from build123d import *

# Parameters (mm, degrees)
ESQUISSE2_R             = 3
ESQUISSE2_R_2           = 1.825
BOSS_EXTRU_1_DEPTH      = 11.5
ESQUISSE3_R             = 10
ENL_V_MAT_EXTRU_1_DEPTH = 4
CONG_1_R                = 5
FILLET1_R               = 5


with BuildPart() as part:
    # Esquisse2 → Boss.-Extru.1 (new body)
    # profile 1 of 4: a face of its own
    with BuildSketch(Plane.XY):
        with Locations((-10, 5)):
            Circle(ESQUISSE2_R)
        with Locations((-10, 5)):
            Circle(ESQUISSE2_R_2, mode=Mode.SUBTRACT)
    # profile 2 of 4: a face of its own
    with BuildSketch(Plane.XY):
        with Locations((10, 5)):
            Circle(ESQUISSE2_R)
        with Locations((10, 5)):
            Circle(ESQUISSE2_R_2, mode=Mode.SUBTRACT)
    # profile 3 of 4: a face of its own
    with BuildSketch(Plane.XY):
        with Locations((0, -6.825)):
            Circle(ESQUISSE2_R)
        with Locations((0, -6.825)):
            Circle(ESQUISSE2_R_2, mode=Mode.SUBTRACT)
    # profile 4 of 4: a face of its own
    with BuildSketch(Plane.XY):
        Polygon((-8.175, 5), (8.175, 5), (0, -5), align=None)
    extrude(amount=BOSS_EXTRU_1_DEPTH)

    # Esquisse3 → Enlèv. mat.-Extru.1 (cut)
    with BuildSketch(Plane.XY.offset(3.75)):
        with Locations((10, 5)):
            Circle(ESQUISSE3_R)
    extrude(amount=ENL_V_MAT_EXTRU_1_DEPTH, mode=Mode.SUBTRACT)

    # Congé1
    # the kernel refuses this fillet: 5 mm, written as the material it adds along each edge
    with BuildSketch(Plane(origin=(-7, 5, 0), x_dir=(-0.3311912213512006, 0.9435636570469954, 0), z_dir=(0, 0, 1))) as cong_1_piece_1:
        with BuildLine():
            CenterArc((3.643103435, -4.717818285), CONG_1_R, 109.341093727, 51.317812547)
            Line((-1.07471485, -3.061862178), (0, 0))
            ThreePointArc((0, 0), (0.993573664, -0.169309029), (1.987147328, 0))
        make_face()
    extrude(amount=11.5)
    with BuildSketch(Plane(origin=(-7.231093941, 3.845374851, 11.5), x_dir=(-0.7661000074497634, -0.6427213848826507, 0), z_dir=(0, 0, -1))) as cong_1_piece_2:
        with BuildLine():
            CenterArc((5.056907819, -4.440322454), CONG_1_R, 117.368969646, 63.360078756)
            Line((0.057312583, -4.503942212), (0, 0))
            ThreePointArc((0, 0), (1.379156678, -0.335806528), (2.758313356, 0))
        make_face()
    extrude(amount=11.5)
    with BuildSketch(Plane(origin=(-0.858096974, -3.950340093, 11.5), x_dir=(-0.6329215353519139, 0.7742159453846039, 0), z_dir=(0, 0, -1))) as cong_1_piece_3:
        with BuildLine():
            CenterArc((4.246739065, -5), CONG_1_R, 90, 61.27443838)
            ThreePointArc((-0.137920096, -2.596926126), (0.227062491, -1.314184518), (0, 0))
            Line((0, 0), (4.246739065, 0))
        make_face()
    extrude(amount=11.5)
    with BuildSketch(Plane(origin=(7.231093941, 3.845374851, 11.5), x_dir=(-0.6329215353519138, -0.774215945384604, 0), z_dir=(0, 0, -1))) as cong_1_piece_4:
        with BuildLine():
            CenterArc((4.504306848, -5), CONG_1_R, 90, 63.360078756)
            ThreePointArc((0.035096646, -2.758090063), (0.353327666, -1.374772245), (0, 0))
            Line((0, 0), (4.504306848, 0))
        make_face()
    extrude(amount=3.75)
    with BuildSketch(Plane(origin=(7, 5, 11.5), x_dir=(-1, 0, 0), z_dir=(0, 0, -1))) as cong_1_piece_5:
        with BuildLine():
            CenterArc((3.244997998, 5), CONG_1_R, 218.682187453, 51.317812547)
            ThreePointArc((-0.658125751, 1.875), (-0.169309029, 0.993573664), (0, 0))
            Line((0, 0), (3.244997998, 0))
        make_face()
    extrude(amount=3.75)
    with BuildSketch(Plane(origin=(0.858096974, -3.950340093, 11.5), x_dir=(0.7395598752725667, -0.6730907746261462, 0), z_dir=(0, 0, -1))) as cong_1_piece_6_section:
        with BuildLine():
            CenterArc((4.767740899, -4.505933799), CONG_1_R, 115.685497342, 61.27443838)
            Line((-0.225222573, -4.240762606), (0, 0))
            ThreePointArc((0, 0), (1.300292973, -0.29643972), (2.600585945, 0))
        make_face()
    cong_1_piece_6 = extrude(amount=11.5, mode=Mode.PRIVATE)
    cong_1_piece_6 = cong_1_piece_6 - Plane(origin=(10, 5, 9.625), x_dir=(1, 0, 0), z_dir=(0, 0, -1)) * Cylinder(10, 40, mode=Mode.PRIVATE)
    add(cong_1_piece_6)
    with BuildSketch(Plane(origin=(0.858096974, -3.950340093, 11.5), x_dir=(0.7395598752725667, -0.6730907746261462, 0), z_dir=(0, 0, -1))) as cong_1_piece_7_section:
        with BuildLine():
            CenterArc((4.767740899, -4.505933799), CONG_1_R, 115.685497342, 61.27443838)
            Line((-0.225222573, -4.240762606), (0, 0))
            ThreePointArc((0, 0), (1.300292973, -0.29643972), (2.600585945, 0))
        make_face()
    cong_1_piece_7 = extrude(amount=22.116847663, mode=Mode.PRIVATE)
    cong_1_piece_7 = split(cong_1_piece_7, bisect_by=Plane(origin=(2.909028405, -1.544063306, 7.75), z_dir=(0, 0, 1)), keep=Keep.TOP, mode=Mode.PRIVATE)
    add(cong_1_piece_7)
    with BuildSketch(Plane(origin=(0.858096974, -3.950340093, 22.116847663), x_dir=(0.7395598752725666, -0.6730907746261463, 0), z_dir=(0, 0, -1))) as cong_1_piece_8_section:
        with BuildLine():
            CenterArc((4.767740899, -4.505933799), CONG_1_R, 115.685497342, 61.27443838)
            Line((-0.225222573, -4.240762606), (0, 0))
            ThreePointArc((0, 0), (1.300292973, -0.29643972), (2.600585945, 0))
        make_face()
    cong_1_piece_8 = extrude(amount=22.116847663, mode=Mode.PRIVATE)
    cong_1_piece_8 = split(cong_1_piece_8, bisect_by=Plane(origin=(2.909028405, -1.544063306, 3.75), z_dir=(0, 0, -1)), keep=Keep.TOP, mode=Mode.PRIVATE)
    add(cong_1_piece_8)

    # Fillet1
    fillet1_edges = [part.edges().sort_by_distance(p)[0] for p in [
        (7.231093941, 3.845374851, 1.875),
        (7, 5, 1.875),
    ]]
    fillet(fillet1_edges, radius=FILLET1_R)


solid = part.part
The listing builds one solid part. Answer for the finished solid, in the listing's coordinates (mm). A direction names the side the tool comes from. Round coordinates to 2 decimals unless told otherwise and drop trailing zeros. Order: outer loops, then holes, each group sorted by start corner. A loop starts at its lowest first (then second) coordinate and runs counter-clockwise, first axis right, second up. Notation, with made-up numbers: M 57,1.5 L 77,1.5 A26 cw 77,19.5 Z; hole C -17,59 d1. An arc over 180 degrees is marked long. Answer in a Markdown table with one row per item. Add a question column.
1) The part is cut by section D-D on x = 5.75. Determine the outline of the cut face in (y, z).
2) Which of the six approach directions +Z, -Z, +X, -X, +Y, -Y give full straight-line access (tool end or side, diameter ignored) to faces 4 (the face through (5.948, 5.507, 9.651)), 5 (the face through (6.656, 1.932, 1.849)), 6 (the face through (6, 3, 7.75))?
3) The part is cut by section A-A on x = 10. Determine the outline of the cut face in (y, z) (3 decimals).
4) Determine the mould class of faces 1 (the face through (5, 3, 3.75)), 2 (the face through (3.969, -0.145, 9.599)), 3 (the face through (-2.48, -3.04, 5.83)) for opening direction Y: pulls with the +Y half, pulls with the -Y half, needs draft (parallel to the pull), parting line crosses it, or undercut.
5) Flat-ended cylindrical pins translate along their axes: pin 1 Ø3.5 at (x, y) = (10, 5) entering from -Z; pin 2 Ø3 at (x, z) = (-1.5, 8.5) entering from +Y; pin 3 Ø4 at (x, z) = (-3, 3) entering from -Y; pin 4 Ø6 at (x, z) = (-1.5, 3.5) entering from +Y. Find the tip coordinate at first contact, or state that the pin passes through.
6) The part is cut by section B-B on y = 6.25. Determine the outline of the cut face in (x, z).
7) The part is cut by section C-C on z = 9.25. Determine the outline of the cut face in (x, y) (3 decimals), plus the area to 3 significant figures.
8) Consider line 1 along Z through (x, y) = (3.75, 3.5); line 2 along Y through (x, z) = (10, 9.2) (3 decimals); line 3 along X through (y, z) = (6.5, 8). Determine where each line is inside the solid, lowest interval first. Write a range as from..to.
Findings below:
| question | item | result |
|---|---|---|
| 1 | outline | M 1.52,0 L 5.42,0 L 5.42,3.75 L 1.52,3.75 Z; M 1.52,7.75 L 5.42,7.75 L 5.42,11.5 L 1.52,11.5 Z |
| 2 | face 4 | +Z, -Z, +Y |
| 2 | face 5 | +Z, -Z, -Y |
| 2 | face 6 | +X, +Y |
| 3 | outline | M 2,0 L 3.175,0 L 3.175,3.75 L 2,3.75 Z; M 2,7.75 L 3.175,7.75 L 3.175,11.5 L 2,11.5 Z; M 6.825,0 L 8,0 L 8,3.75 L 6.825,3.75 Z; M 6.825,7.75 L 8,7.75 L 8,11.5 L 6.825,11.5 Z |
| 4 | face 1 | needs draft |
| 4 | face 2 | pulls with the -Y half |
| 4 | face 3 | undercut |
| 5 | pin 1 | passes through |
| 5 | pin 2 | stops at y = 5 |
| 5 | pin 3 | stops at y = -9.65 |
| 5 | pin 4 | stops at y = 5.06 |
| 6 | outline | M -12.73,0 L -11.33,0 L -11.33,11.5 L -12.73,11.5 Z; M -8.67,0 L -7.06,0 L -7.06,11.5 L -8.67,11.5 Z; M 7.06,0 L 8.67,0 L 8.67,3.75 L 7.06,3.75 Z; M 7.06,7.75 L 8.67,7.75 L 8.67,11.5 L 7.06,11.5 Z; M 11.33,0 L 12.73,0 L 12.73,3.75 L 11.33,3.75 Z; M 11.33,7.75 L 12.73,7.75 L 12.73,11.5 L 11.33,11.5 Z |
| 7 | outline | M -9.344,2.073 A5 cw -4.38,0.358 L -3.546,-0.662 A5 cw -2.781,-5.701 A3 ccw long 2.781,-5.701 A5 cw 3.546,-0.662 L 4.38,0.358 A5 cw 9.344,2.073 A3 ccw long 7.658,6.875 A5 cw 3.755,5 L -3.755,5 A5 cw -7.658,6.875 A3 ccw long Z; hole C -10,5 d3.65; hole C 0,-6.825 d3.65; hole C 10,5 d3.65 |
| 7 | area | 146 mm² |
| 8 | line 1 | z = 0..3.75, 7.75..11.5 |
| 8 | line 2 | y = 2..3.175, 6.825..8 |
| 8 | line 3 | x = -12.6..-11.04, -8.96..-7.33, 7.33..8.96, 11.04..12.6 |
